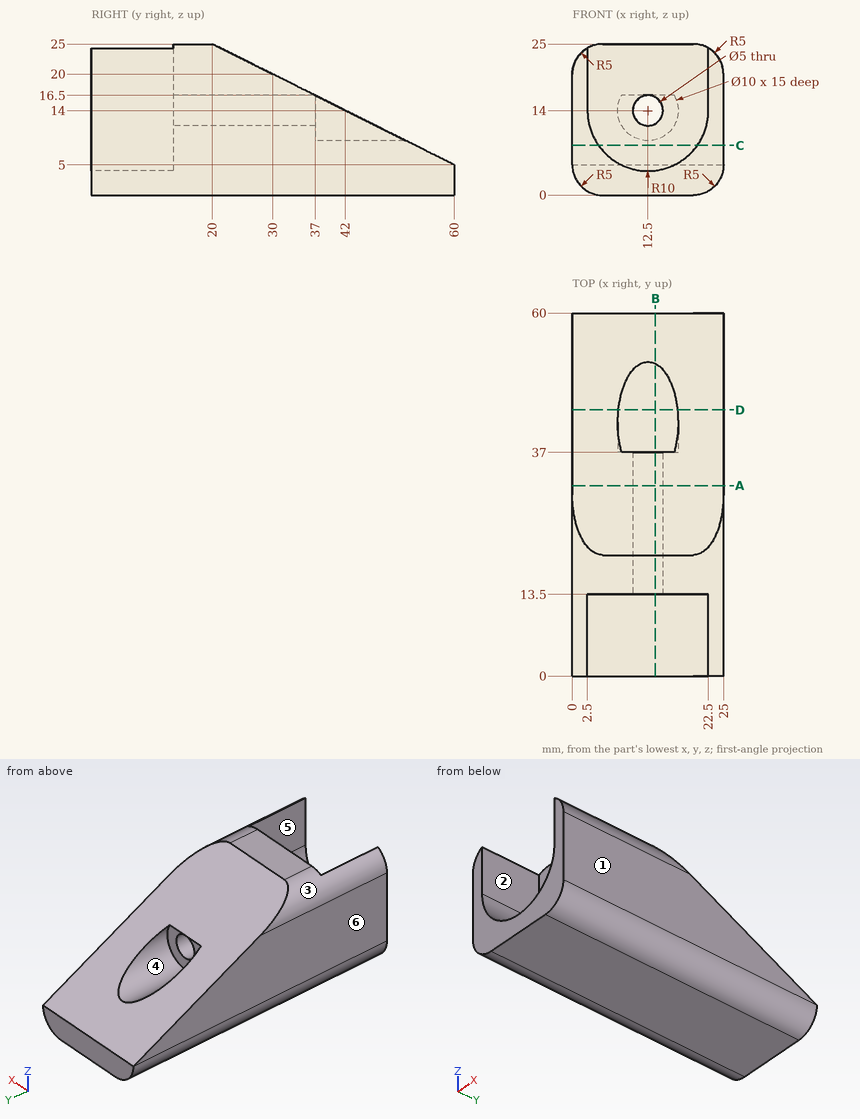
Print and shaded views of the part. All mm, measured from the part's lowest x, y and z. A direction names the side the tool comes from. Give positions to 0.01 mm unless a question says otherwise; leave off trailing zeros. Loops run counter-clockwise (first coordinate to the right, second up) from the corner with the lowest first, then second, coordinate; pieces in that order, holes last. Notation, with made-up numbers: (58, 44) -> (94, 44) arc R24 cw to (94, 70) -> close; hole circle Ø5 at (-12, -16). An arc over 180 degrees is marked (long way). Use CSV: the item, a comma, the result in double quotes. Start each with the question number.
1) Slice it at A-A on y = 31.5. Give the cut face in (x, z).
2) Tool access for the marked faces 4, 5 and 6: list every direction of +Z, -Z, +X, -X, +Y, -Y with a clear straight run to the whole face (end or side of a thin tool).
3) Slice it at D-D on y = 44. Give the cut face in (x, z).
4) Mould opens along X. For the marked faces 1, 2 and 3 say: released by +X, released by -X, zero draft, split by the parting line, or undercut.
5) Slice it at B-B on x = 13.75. Give the cut face in (y, z).
6) Flat gauge pins, fed straight in: pin 1 Ø4 at (x, y) = (9.5, 37) entering from +Z; pin 2 Ø8 at (x, z) = (11.5, 13) entering from +Y; pin 3 Ø4 at (x, y) = (15, 49.5) entering from +Z. Where does each tip first touch, or does it go through?
7) Wall check: line 1 (X direction, y = 21.75, z = 14); line 2 (Z direction, x = 12.5, y = 19); line 3 (X direction, y = 13, z = 16). Give the ranges that are in metal, low to high.
8) Slice it at C-C on z = 8.25. Give the cut face in (x, y).
Computed values:
1,outline,"(0, 5) arc R5 ccw to (5, 0) -> (20, 0) arc R5 ccw to (25, 5) -> (25, 19.25) -> (0, 19.25) -> close; hole circle Ø5 at (12.5, 14)"
2,face 4,"+Y"
2,face 5,"+Z, -Y"
2,face 6,"+Z, -Z, -X, +Y, -Y"
3,outline,"(0, 5) arc R5 ccw to (5, 0) -> (20, 0) arc R5 ccw to (25, 5) -> (25, 13) -> (17.4, 13) arc R5 cw to (7.6, 13) -> (0, 13) -> close"
4,face 1,"released by +X"
4,face 2,"undercut"
4,face 3,"released by -X"
5,outline,"(0, 0) -> (60, 0) -> (60, 5) -> (51.68, 9.16) -> (37, 9.16) -> (37, 11.83) -> (13.5, 11.83) -> (13.5, 4.08) -> (0, 4.08) -> close; (13.5, 16.17) -> (37, 16.17) -> (37, 16.5) -> (20, 25) -> (13.5, 25) -> close"
6,pin 1,"stops at z = 17.5"
6,pin 2,"stops at y = 52"
6,pin 3,"stops at z = 10.94"
7,line 1,"x = 0 to 10, 15 to 25"
7,line 2,"z = 0 to 11.5, 16.5 to 25"
7,line 3,"x = 0 to 2.5, 22.5 to 25"
8,outline,"(0, 0) -> (4.32, 0) -> (4.32, 13.5) -> (20.68, 13.5) -> (20.68, 0) -> (25, 0) -> (25, 53.5) -> (0, 53.5) -> close"
